Read the model definition and answer for the solid it produces. Units are mm, in the model's axes. A direction names the side the tool comes from. Give positions to 0.01 mm unless a question says otherwise; leave off trailing zeros. Write each loop counter-clockwise with the first axis right and the second up, starting at its lowest first coordinate (ties: lowest second). Pieces come first, ordered by that corner, then holes. Notation, with made-up numbers: M 85.25,7.5 L 134.25,7.5 A15 cw 134.25,21.5 Z; hole C -15,-26.5 d11. An arc over 180 degrees is marked long. Put each result on its own line as item: value.
from build123d import *

# Parameters (mm, degrees)
SKETCH_1_R          = 7
EXTRUDE_1_DEPTH     = 85
SKETCH_2_R          = 7.5
SKETCH_2_R_2        = 6
CUT_EXTRUDE_1_DEPTH = 12


with BuildPart() as part:
    # 草图1 → 凸台-拉伸1 (new body)
    with BuildSketch(Plane(origin=(0, 0, 0), x_dir=(0, 0, -1), z_dir=(1, 0, 0))):
        Circle(SKETCH_1_R)
    extrude(amount=EXTRUDE_1_DEPTH)

    # 草图2 → 切除-拉伸1 (cut)
    with BuildSketch(Plane.ZY):
        Circle(SKETCH_2_R)
        Circle(SKETCH_2_R_2, mode=Mode.SUBTRACT)
    cut_extrude_1 = extrude(amount=-CUT_EXTRUDE_1_DEPTH, mode=Mode.SUBTRACT)

    # 镜向1: 切除-拉伸1 across plane
    add(cut_extrude_1.mirror(Plane(origin=(42.5, 0, 0), x_dir=(0, 0, 1), z_dir=(1, 0, 0))), mode=Mode.SUBTRACT)


solid = part.part
(1) Section A-A on z = 0 is taken. Determine the outline of the cut face in (x, y), and give its area (3 significant figures).
Result:
outline: M 0,-6 L 12,-6 L 12,-7 L 73,-7 L 73,-6 L 85,-6 L 85,6 L 73,6 L 73,7 L 12,7 L 12,6 L 0,6 Z
area: 1,140 mm²
(2) Section D-D on x = 5 is taken. Determine the outline of the cut face in (y, z), and give its area (3 significant figures).
Result:
outline: C 0,0 d12
area: 113 mm²
(3) Section B-B on x = 50 is taken. Determine the outline of the cut face in (y, z).
Result:
outline: C 0,0 d14
(4) Straight lines are drawn through the part: line 1 along X through (y, z) = (5.25, -4); line 2 along Y through (x, z) = (19.5, -0.25). For each, find the intervals that lie inside material, in ascending order. Write a range as from..to.
Result:
line 1: x = 12..73
line 2: y = -7..7
(5) Given pin 1 Ø7 at (y, z) = (0, 0) entering from -X; pin 2 Ø1 at (x, y) = (24, -1.5) entering from +Z; pin 3 Ø1.5 at (x, y) = (33, -1) entering from +Z; pin 4 Ø8 at (x, y) = (45.5, -4.5) entering from -Z, each flat-ended and moving along its own axis, determine where each tip first touches the part or whether it passes through.
Result:
pin 1: stops at x = 0
pin 2: stops at z = 6.93
pin 3: stops at z = 7
pin 4: stops at z = -6.98
(6) Section C-C on y = -1 is taken. Determine the outline of the cut face in (x, z).
Result:
outline: M 0,-5.92 L 12,-5.92 L 12,-6.93 L 73,-6.93 L 73,-5.92 L 85,-5.92 L 85,5.92 L 73,5.92 L 73,6.93 L 12,6.93 L 12,5.92 L 0,5.92 Z
(7) Which of the six approach directions +Z, -Z, +X, -X, +Y, -Y give full straight-line access (tool end or side, diameter ignored) to faces 1 (the face through (6, 0, -6)), 2 (the face through (85, 0, 0)), 3 (the face through (79, 0, -6))?
Result:
face 1: -X
face 2: +Z, -Z, +X, +Y, -Y
face 3: +X
